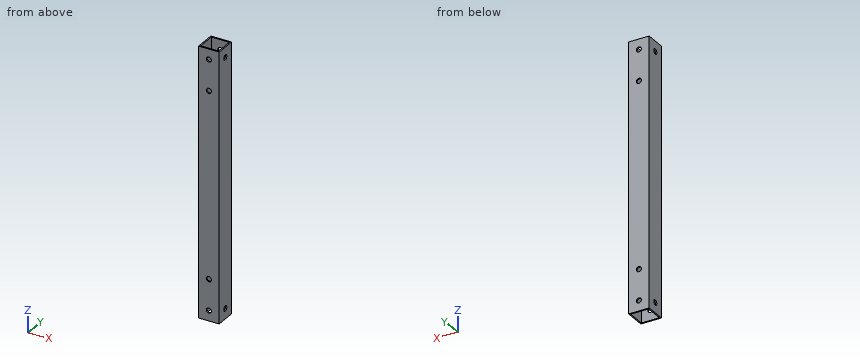
Autodesk Inventor part; units mm, degrees
ref_plane "YZ Plane" through (0, 0, 0) normal (1, 0, 0) x (0, 1, 0)
ref_plane "XZ Plane" through (0, 0, 0) normal (0, 1, 0) x (-1, 0, 0)
ref_plane "XY Plane" through (0, 0, 0) normal (0, 0, 1) x (1, 0, 0)
sketch "Sketch1" plane through (0, 0, 0) normal (0, 0, 1) x (1, 0, 0)
  line L0 (0, 0) -> (25.4, 0)
  line L1 (25.4, 0) -> (25.4, 25.4)
  line L2 (25.4, 25.4) -> (0, 25.4)
  line L3 (0, 25.4) -> (0, 0)
  line L4 (1.5875, 23.8125) -> (23.8125, 23.8125)
  line L5 (23.8125, 23.8125) -> (23.8125, 1.5875)
  line L6 (23.8125, 1.5875) -> (1.5875, 1.5875)
  line L7 (1.5875, 1.5875) -> (1.5875, 23.8125)
  dimension "d0" = 25.4
  dimension "d1" = 25.4
  dimension "d2" = 1.5875
extrude "Extrusion1" add sketch "Sketch1" against normal blind 330.2
sketch "Sketch2" plane through (0, 0, 0) normal (0, -1, 0) x (1, 0, 0)
  line L0 (0, -330.2) -> (25.4, -330.2)
  point P0 (12.7, -317.5)
  point P1 (12.7, -279.4)
  dimension "d5" = 38.1
  dimension "d6" = 12.7
hole "Hole1" at (12.7, 0, -317.5) at (12.7, 0, -279.4) direction (0, 1, 0) diameter 6.35 depth 25.4 tip angle 118
sketch "Sketch3" plane through (0, 25.4, 0) normal (0, 1, 0) x (1, 0, 0)
  line L0 (0, 0) -> (0, 330.2)
  line L1 (25.4, 0) -> (0, 0)
  point P0 (12.7, 12.7)
  dimension "d25" = 12.7
  dimension "d26" = 12.7
sketch "Sketch4" plane through (25.4, 0, 0) normal (1, 0, 0) x (0, 0, -1)
  line L0 (330.2, 0) -> (330.2, 25.4)
  line L1 (0, 25.4) -> (330.2, 25.4)
  line L2 (0, 0) -> (0, 25.4)
  point P0 (317.5, 12.7)
  point P1 (12.7, 12.7)
  dimension "d14" = 12.7
  dimension "d15" = 12.7
  dimension "d16" = 12.7
  dimension "d17" = 12.7
hole "Hole2" at (25.4, 12.7, -12.7) at (25.4, 12.7, -317.5) direction (-1, 0, 0) diameter 6.35 depth 25.4 tip angle 118
hole "Hole3" at (12.7, 25.4, -12.7) direction (0, -1, 0) diameter 6.35 depth 25.4 tip angle 118
sketch "Sketch5" plane through (0, 25.4, 0) normal (0, 1, 0) x (1, 0, 0)
  line L0 (25.4, 0) -> (0, 0)
  point P0 (12.7, 50.8)
  dimension "d34" = 50.8
hole "Hole4" at (12.7, 25.4, -50.8) direction (0, -1, 0) diameter 6.35 depth 50.8 tip angle 118
properties part number "1tube_13_layer2_side"
Model file for the job. Use its own axes, mm. Round coordinates to 2 decimals unless told otherwise and drop trailing zeros. Write each loop counter-clockwise with the first axis right and the second up, starting at its lowest first coordinate (ties: lowest second). Pieces come first, ordered by that corner, then holes. Notation, with made-up numbers: M -39.75,1 L -19.75,1 A20 ccw -19.75,18 Z; hole C 53,33.5 d7. An arc over 180 degrees is marked long. Put each result on its own line as item: value.
Item 1: Cut at A-A (y = 12.7). List the corners of the cut face in (x, z) (1 decimal), and give its area (3 significant figures).
Responses:
outline: M 0,-330.2 L 1.6,-330.2 L 1.6,-320.7 L 0,-320.7 Z; M 0,-314.3 L 1.6,-314.3 L 1.6,-15.9 L 0,-15.9 Z; M 0,-9.5 L 1.6,-9.5 L 1.6,0 L 0,0 Z; M 23.8,-330.2 L 25.4,-330.2 L 25.4,-320.7 L 23.8,-320.7 Z; M 23.8,-314.3 L 25.4,-314.3 L 25.4,-15.9 L 23.8,-15.9 Z; M 23.8,-9.5 L 25.4,-9.5 L 25.4,0 L 23.8,0 Z
area: 1,010 mm²
Item 2: Cut at D-D (z = -12.7). List the corners of the cut face in (x, y) (1 decimal).
Responses:
outline: M 0,0 L 9.5,0 L 9.5,1.6 L 1.6,1.6 L 1.6,9.5 L 0,9.5 Z; M 0,15.9 L 1.6,15.9 L 1.6,23.8 L 9.5,23.8 L 9.5,25.4 L 0,25.4 Z; M 15.9,0 L 25.4,0 L 25.4,9.5 L 23.8,9.5 L 23.8,1.6 L 15.9,1.6 Z; M 15.9,23.8 L 23.8,23.8 L 23.8,15.9 L 25.4,15.9 L 25.4,25.4 L 15.9,25.4 Z
Item 3: Cut at C-C (z = -279.4). List the corners of the cut face in (x, y) (1 decimal), and give its area (3 significant figures).
Responses:
outline: M 0,0 L 9.5,0 L 9.5,1.6 L 1.6,1.6 L 1.6,23.8 L 9.5,23.8 L 9.5,25.4 L 0,25.4 Z; M 15.9,0 L 25.4,0 L 25.4,25.4 L 15.9,25.4 L 15.9,23.8 L 23.8,23.8 L 23.8,1.6 L 15.9,1.6 Z
area: 131 mm²
Item 4: Probe L1, parallel to Z at x = 24.9, y = 12.7 (3 decimals); L2, parallel to Z at x = 12.7, y = 25.05 (3 decimals); L3, parallel to X at y = 9.75, z = -139. List the from-to ranges inside material, lowest first. Write a range as from..to.
Responses:
L1: -330.2..-320.675, -314.325..-15.875, -9.525..0
L2: -330.2..-320.675, -314.325..-282.575, -276.225..-53.975, -47.625..-15.875, -9.525..0
L3: 0..1.59, 23.81..25.4
Item 5: Cut at B-B (x = 5.25). List the corners of the cut face in (y, z).
Responses:
outline: M 0,-330.2 L 1.59,-330.2 L 1.59,0 L 0,0 Z; M 23.81,-330.2 L 25.4,-330.2 L 25.4,0 L 23.81,0 Z
